For this review, take the finished solid that the model builds, in its own axes (mm). A direction names the side the tool comes from. Round coordinates to 2 decimals unless told otherwise and drop trailing zeros. Order: outer loops, then holes, each group sorted by start corner. A loop starts at its lowest first (then second) coordinate and runs counter-clockwise, first axis right, second up. Notation, with made-up numbers: M -26,44.25 L -22,44.25 A25 cw -22,63.25 Z; hole C -13,4.5 d10. An arc over 180 degrees is marked long. Put each result on its own line as item: value.
from build123d import *

# Parameters (mm, degrees)
BOX_W        = 65
BOX_H        = 65
BOX_DEPTH    = 65
SKETCH_R     = 19.339319
POCKET_DEPTH = 10
FILLET_R     = 5
FILLET001_R  = 5


with BuildPart() as part:
    # Box → Box (new body)
    with BuildSketch(Plane.XY):
        with Locations((32.5, 32.5)):
            Rectangle(BOX_W, BOX_H)
    extrude(amount=BOX_DEPTH)

    # Sketch → Pocket (cut)
    with BuildSketch(Plane.YZ.offset(65)):
        with Locations((32.5, 32.5)):
            Circle(SKETCH_R)
    extrude(amount=-POCKET_DEPTH, mode=Mode.SUBTRACT)

    # Fillet
    fillet_edges = [part.edges().sort_by_distance(p)[0] for p in [
        (65, 13.160681, 32.5),
    ]]
    fillet(fillet_edges, radius=FILLET_R)

    # Fillet001
    fillet001_edges = [part.edges().sort_by_distance(p)[0] for p in [
        (32.5, 0, 65),
        (32.5, 65, 65),
        (65, 32.5, 65),
        (0, 32.5, 65),
    ]]
    fillet(fillet001_edges, radius=FILLET001_R)


solid = part.part
(1) Insertion check: pin 1 Ø3 at (y, z) = (34, 33.5) entering from +X; pin 2 Ø5 at (y, z) = (6.5, 58) entering from -X. Each pin has a flat end and moves straight along its axis. Give the tip position at first contact, or say it passes through.
A:
pin 1: stops at x = 55
pin 2: stops at x = 0
(2) To check wall thickness, follow L1, parallel to Z at x = 58.25, y = 32.5; L2, parallel to Y at x = 58, z = 32; L3, parallel to Z at x = 58, y = 15.5. State the ranges of each line that lie inside material, in increasing order.
A:
L1: z = 0 to 13.16, 51.84 to 65
L2: y = 0 to 13.17, 51.83 to 65
L3: z = 0 to 23.28, 41.72 to 65
(3) Add section B-B on z = 32.5. Give the boundary of the cut face in (x, y), then the cut area to 3 significant figures.
A:
outline: M 0,0 L 65,0 L 65,8.16 A5 ccw 60,13.16 L 55,13.16 L 55,51.84 L 60,51.84 A5 ccw 65,56.84 L 65,65 L 0,65 Z
area: 3,830 mm2
(4) For faces 1 (the face through (55, 32, 33)), 2 (the face through (32, 33, 0)), list the 3-axis set-ups (+Z, -Z, +X, -X, +Y, -Y) from which the entire face can be reached by the end or side of a thin tool; tool diameter is ignored.
A:
face 1: +X
face 2: -Z, +X, -X, +Y, -Y
(5) Add section A-A on y = 32.5. Give the boundary of the cut face in (x, z), then the cut area to 3 significant figures.
A:
outline: M 0,0 L 65,0 L 65,8.16 A5 ccw 60,13.16 L 55,13.16 L 55,51.84 L 60,51.84 A5 ccw 65,56.84 L 65,60 A5 ccw 60,65 L 5,65 A5 ccw 0,60 Z
area: 3,820 mm2
(6) Draft analysis for pull direction Y (two halves, no side actions). For faces 3 (the face through (57.535, 29.982, 51.675)), 4 (the face through (33, 63, 64)), 5 (the face through (65, 18, 10)), state which applies: released by +Y, released by -Y, zero draft, split by the parting line, or undercut.
A:
face 3: undercut
face 4: released by +Y
face 5: zero draft
